from build123d import *

# Parameters (mm, degrees)
F2_R      = 6.35
F3_DEPTH  = 59.182
F4_R      = 6.35
F5_DEPTH  = 25.4
F6_R      = 6.35
F7_DEPTH  = 25.4
F8_R      = 6.35
F9_DEPTH  = 39.116
F10_R     = 6.35
F11_DEPTH = 44.45
F12_R     = 6.35
F13_DEPTH = 41.148


with BuildPart() as f1:
    # F0 (on Top) → F1 (revolve)
    with BuildSketch(Plane.XY):
        with BuildLine():
            Line((0, -19.05), (0, -25.4))
            ThreePointArc((0, -25.4), (25.4, 0), (0, 25.4))
            Line((0, 25.4), (0, 19.05))
            ThreePointArc((0, 19.05), (19.05, 0), (0, -19.05))
        make_face()
    revolve(axis=Axis((0, 22.225, 0), (0, -1, 0)))

    # F2 (on Top) → F3 (cut)
    with BuildSketch(Plane.XY):
        Circle(F2_R)
    extrude(amount=-F3_DEPTH, mode=Mode.SUBTRACT)

    # F4 (on Right) → F5 (cut)
    with BuildSketch(Plane.YZ):
        Circle(F4_R)
    extrude(amount=-F5_DEPTH, mode=Mode.SUBTRACT)

    # F6 (on Front) → F7 (cut)
    with BuildSketch(Plane.XZ):
        Circle(F6_R)
    extrude(amount=-F7_DEPTH, mode=Mode.SUBTRACT)

    # F8 (on Right) → F9 (cut)
    with BuildSketch(Plane.YZ):
        Circle(F8_R)
    extrude(amount=F9_DEPTH, mode=Mode.SUBTRACT)

    # F10 (on Front) → F11 (cut)
    with BuildSketch(Plane.XZ):
        Circle(F10_R)
    extrude(amount=F11_DEPTH, mode=Mode.SUBTRACT)

    # F12 (on Top) → F13 (cut)
    with BuildSketch(Plane.XY):
        Circle(F12_R)
    extrude(amount=F13_DEPTH, mode=Mode.SUBTRACT)


solid = f1.part
Geometry: final body of the model. Coordinates: model frame, mm. Give positions to 0.01 mm unless a question says otherwise; leave off trailing zeros. Write each loop counter-clockwise with the first axis right and the second up, starting at its lowest first coordinate (ties: lowest second). Pieces come first, ordered by that corner, then holes. Notation, with made-up numbers: (36.25, 65) - (76.25, 65) arc R26 cw to (76.25, 90) - close; hole circle Ø9 at (24.5, 47). An arc over 180 degrees is marked (long way). Return JSON: item names as keys, results as strings. Group by question number.
1) Section C-C on y = -14.5. Return the cut outline in (x, z), plus the area to 3 significant figures.
2) First-contact query: P1, Ø12, axis at y = -5.5, z = -18, coming from the -X side; P2, Ø1.5, axis at x = 16.5, y = 11.5, coming from the +Z side; P3, Ø2, axis at x = 13.5, y = 6.5, coming from the +Z side. Flat tips, straight axial feed; report the tip coordinate or a pass-through.
3) Section A-A on z = 0. Return the cut outline in (x, y).
4) Mould query, pull axis Z, two halves, no side actions, for faces 1 (the cylindrical face through (-5.04, 21.23, -3.86)), 2 (the cylindrical face through (-1.38, -6.2, 21.23)), 3 (the cylindrical face through (-1.38, -21.23, -6.2)). Classes: released by +Z, released by -Z, zero draft, split by the parting line, or undercut.
5) Section D-D on x = -16. Return the cut outline in (y, z), plus the area to 3 significant figures.
6) Line query: line 1 (Z direction, x = 20.75, y = 0); line 2 (Z direction, x = 8.5, y = 9); line 3 (Y direction, x = 0, z = 20). Output: solid intervals per line, ascending.
Filled in:
{
 "1": {"outline": "circle Ø41.71 at (0, 0); hole circle Ø24.71 at (0, 0)", "area": "887 mm^2"},
 "2": {"P1": "stops at x = -21.93", "P2": "stops at z = 16.44", "P3": "stops at z = 21.2"},
 "3": {"outline": "(-24.59, -6.35) arc R25.4 ccw to (-6.35, -24.59) - (-6.35, -17.96) arc R19.05 cw to (-17.96, -6.35) - close; (-24.59, 6.35) - (-17.96, 6.35) arc R19.05 cw to (-6.35, 17.96) - (-6.35, 24.59) arc R25.4 ccw to start; (6.35, -24.59) arc R25.4 ccw to (24.59, -6.35) - (17.96, -6.35) arc R19.05 cw to (6.35, -17.96) - close; (6.35, 17.96) arc R19.05 cw to (17.96, 6.35) - (24.59, 6.35) arc R25.4 ccw to (6.35, 24.59) - close"},
 "4": {"face 1": "undercut", "face 2": "zero draft", "face 3": "undercut"},
 "5": {"outline": "circle Ø39.45 at (0, 0); hole circle Ø20.68 at (0, 0)", "area": "887 mm^2"},
 "6": {"line 1": "z = -14.65 to -6.35, 6.35 to 14.65", "line 2": "z = -22.18 to -14.48, 14.48 to 22.18", "line 3": "y = -15.66 to -6.35, 6.35 to 15.66"}
}
